from build123d import *

# Parameters (mm, degrees)
F0_W          = 75
F0_H          = 75
F1_DEPTH      = 4
F2_W          = 75
F2_H          = 75
F2_W_2        = 69
F2_H_2        = 69
F3_DEPTH      = 12
F5_DEPTH      = 25
F6_R          = 0.75
F7_DEPTH      = 25
F7_DEPTH_BACK = 72.001
F8_R          = 0.75
F9_DEPTH      = 25
F9_DEPTH_BACK = 72.001


with BuildPart() as f1:
    # F0 (on Top) → F1 (new body)
    with BuildSketch(Plane.XY):
        with Locations((37.5, 37.5)):
            Rectangle(F0_W, F0_H)
    extrude(amount=F1_DEPTH)

    # F2 (on face) → F3 (join)
    with BuildSketch(Plane.XY.offset(4)):
        with Locations((37.5, 37.5)):
            Rectangle(F2_W, F2_H)
        with Locations((37.5, 37.5)):
            Rectangle(F2_W_2, F2_H_2, mode=Mode.SUBTRACT)
    extrude(amount=F3_DEPTH)

    # F4 (on face) → F5 (cut)
    with BuildSketch(Plane(origin=(0, 0, 0), x_dir=(1, 0, 0), z_dir=(0, 0, -1))):
        with BuildLine():
            ThreePointArc((13.1213203436, -18.6213203436), (9.8519497029, -17.9710020896), (8, -20.7426406871))
            Line((8, -20.7426406871), (8, -54.2573593129))
            ThreePointArc((8, -54.2573593129), (9.8519497029, -57.0289979104), (13.1213203436, -56.3786796564))
            Line((13.1213203436, -56.3786796564), (29.8786796564, -39.6213203436))
            ThreePointArc((29.8786796564, -39.6213203436), (30.7573593129, -37.5), (29.8786796564, -35.3786796564))
            Line((29.8786796564, -35.3786796564), (13.1213203436, -18.6213203436))
        make_face()
        with BuildLine():
            ThreePointArc((35.3786796564, -29.8786796564), (37.5, -30.7573593129), (39.6213203436, -29.8786796564))
            Line((39.6213203436, -29.8786796564), (56.3786796564, -13.1213203436))
            ThreePointArc((56.3786796564, -13.1213203436), (57.0289979104, -9.8519497029), (54.2573593129, -8))
            Line((54.2573593129, -8), (20.7426406871, -8))
            ThreePointArc((20.7426406871, -8), (17.9710020896, -9.8519497029), (18.6213203436, -13.1213203436))
            Line((18.6213203436, -13.1213203436), (35.3786796564, -29.8786796564))
        make_face()
        with BuildLine():
            Line((67, -54.2573593129), (67, -20.7426406871))
            ThreePointArc((67, -20.7426406871), (65.1480502971, -17.9710020896), (61.8786796564, -18.6213203436))
            Line((61.8786796564, -18.6213203436), (45.1213203436, -35.3786796564))
            ThreePointArc((45.1213203436, -35.3786796564), (44.2426406871, -37.5), (45.1213203436, -39.6213203436))
            Line((45.1213203436, -39.6213203436), (61.8786796564, -56.3786796564))
            ThreePointArc((61.8786796564, -56.3786796564), (65.1480502971, -57.0289979104), (67, -54.2573593129))
        make_face()
        with BuildLine():
            Line((56.3786796564, -61.8786796564), (39.6213203436, -45.1213203436))
            ThreePointArc((39.6213203436, -45.1213203436), (37.5, -44.2426406871), (35.3786796564, -45.1213203436))
            Line((35.3786796564, -45.1213203436), (18.6213203436, -61.8786796564))
            ThreePointArc((18.6213203436, -61.8786796564), (17.9710020896, -65.1480502971), (20.7426406871, -67))
            Line((20.7426406871, -67), (54.2573593129, -67))
            ThreePointArc((54.2573593129, -67), (57.0289979104, -65.1480502971), (56.3786796564, -61.8786796564))
        make_face()
    extrude(amount=-F5_DEPTH, mode=Mode.SUBTRACT)

    # F6 (on face) → F7 (cut, two sides)
    with BuildSketch(Plane.XZ.offset(-72)) as f7_sk:
        with Locations((37.5, 10)):
            Circle(F6_R)
    extrude(amount=-F7_DEPTH, mode=Mode.SUBTRACT)
    extrude(f7_sk.sketch, amount=F7_DEPTH_BACK, mode=Mode.SUBTRACT)

    # F8 (on face) → F9 (cut, two sides)
    with BuildSketch(Plane.YZ.offset(3)) as f9_sk:
        with Locations((37.5, 10)):
            Circle(F8_R)
    extrude(amount=-F9_DEPTH, mode=Mode.SUBTRACT)
    extrude(f9_sk.sketch, amount=F9_DEPTH_BACK, mode=Mode.SUBTRACT)


solid = f1.part
The model under review builds one solid part; all positions refer to its coordinate system, in mm. A direction names the side the tool comes from. Give positions to 0.01 mm unless a question says otherwise; leave off trailing zeros. Write each loop counter-clockwise with the first axis right and the second up, starting at its lowest first coordinate (ties: lowest second). Pieces come first, ordered by that corner, then holes. Notation, with made-up numbers: M 48.25,-0.5 L 66.25,-0.5 A18 ccw 66.25,29.5 Z; hole C -33.5,7.25 d8. An arc over 180 degrees is marked long. One line per question, with ' | ' between items. Start each with the question number.
Item 1: We need section A-A on z = 14. Write out the cut boundary in (x, y).
Item 2: For faces 4 (the flat face through (37, 75, 8)), 5 (the flat face through (37, 3, 11)), 6 (the flat face through (37, 67, 2)), list the 3-axis set-ups (+Z, -Z, +X, -X, +Y, -Y) from which the entire face can be reached by the end or side of a thin tool; tool diameter is ignored.
Item 3: For pin 1 (1 mm diameter, centred on x = 19.5, y = 10, fed in from -Z); pin 2 (8 mm diameter, centred on x = 23.5, y = 53.5, fed in from +Z), all flat-tipped, find the tip position at first contact; note any pin that passes through.
Item 4: Draft analysis for pull direction X (two halves, no side actions). For faces 1 (the flat face through (21.6, 27.1, 2)), 2 (the flat face through (75, 37, 8)), 3 (the flat face through (37, 0, 8)), state which applies: released by +X, released by -X, zero draft, split by the parting line, or undercut.
Item 5: Wall thickness on line 1 (X direction, y = 67.5, z = 5.25); line 2 (X direction, y = 56, z = 1.75): over which ranges is each line inside the solid? List them lowest first. Write a range as from..to.
Item 6: We need section D-D on x = 24. Write out the cut boundary in (y, z).
Item 7: We need section B-B on y = 64. Write out the cut boundary in (x, z), plus the area to 3 significant figures.
Item 8: We need section C-C on y = 26. Write out the cut boundary in (x, z).
Results found:
1) outline: M 0,0 L 75,0 L 75,75 L 0,75 Z; hole M 3,3 L 72,3 L 72,72 L 3,72 Z
2) face 4: +Z, -Z, +X, -X, +Y | face 5: +Z | face 6: +Z, -Z
3) pin 1: passes through | pin 2: stops at z = 4
4) face 1: undercut | face 2: released by +X | face 3: zero draft
5) line 1: x = 0..3, 72..75 | line 2: x = 0..8.56, 13.5..24.5, 50.5..61.5, 66.44..75
6) outline: M 0,0 L 8,0 L 8,4 L 3,4 L 3,16 L 0,16 Z; M 18.5,0 L 29.5,0 L 29.5,4 L 18.5,4 Z; M 45.5,0 L 56.5,0 L 56.5,4 L 45.5,4 Z; M 67,0 L 75,0 L 75,16 L 72,16 L 72,4 L 67,4 Z
7) outline: M 0,0 L 17.74,0 L 17.74,4 L 3,4 L 3,16 L 0,16 Z; M 57.26,0 L 75,0 L 75,16 L 72,16 L 72,4 L 57.26,4 Z | area: 214 mm2
8) outline: M 0,0 L 8,0 L 8,4 L 3,4 L 3,16 L 0,16 Z; M 20.5,0 L 31.5,0 L 31.5,4 L 20.5,4 Z; M 43.5,0 L 54.5,0 L 54.5,4 L 43.5,4 Z; M 67,0 L 75,0 L 75,16 L 72,16 L 72,4 L 67,4 Z
